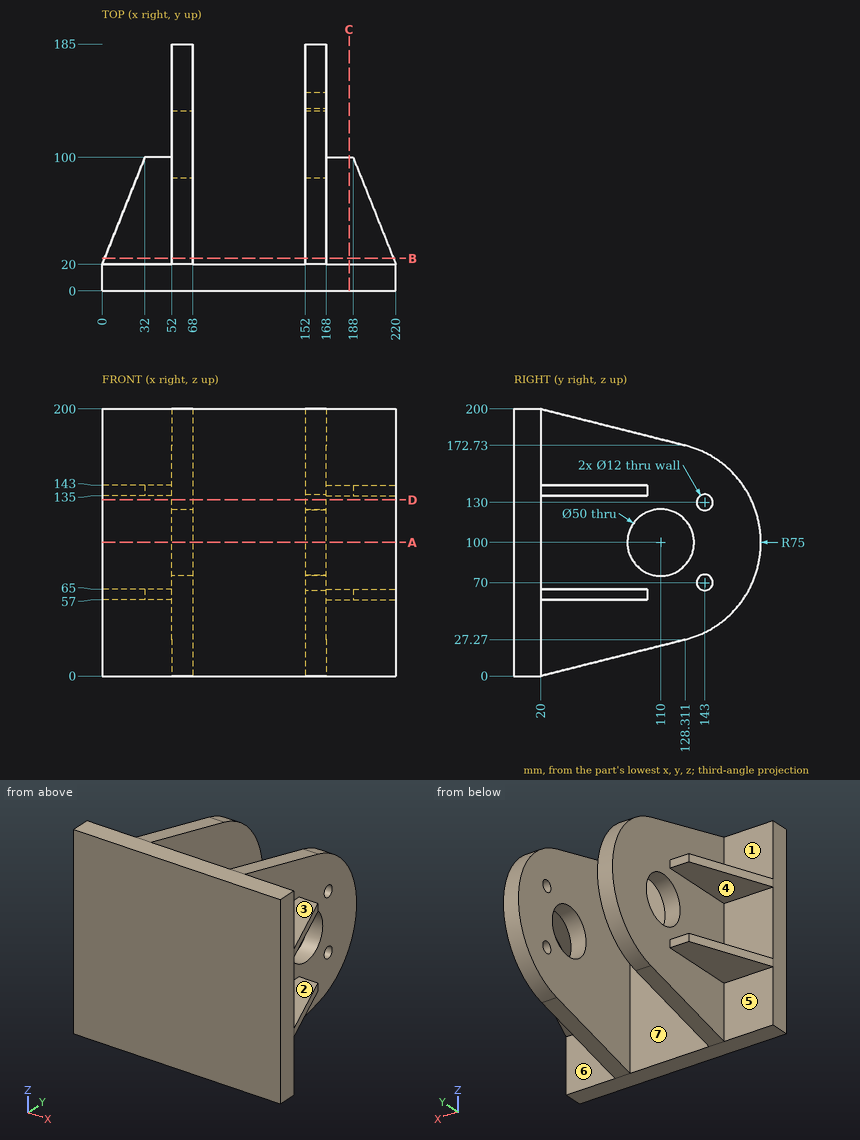
Here's the drawing with two shaded views (mm, measured from the low corner). I have some questions. A direction names the side the tool comes from. Round coordinates to 2 decimals unless told otherwise and drop trailing zeros. Loops run counter-clockwise (first coordinate to the right, second up) from the corner with the lowest first, then second, coordinate; pieces in that order, holes last. Notation, with made-up numbers: (81, -23) -> (138, -23) arc R21 cw to (138, -12) -> close; hole circle Ø8 at (-34.75, -8). An arc over 180 degrees is marked (long way). Answer as CSV lines item,"result". Start each with the question number.
1. Imagine slicing it at D-D on z = 132. Write out the boundary of the cut face in (x, y).
2. Imagine slicing it at A-A on z = 100. Write out the boundary of the cut face in (x, y), plus the area to 3 significant figures.
3. For the marked faces 1, 2, 3, 4 and 5, which set-ups out of +Z, -Z, +X, -X, +Y, -Y let a thin tool reach every point of the face, with its end or its side?
4. Imagine slicing it at C-C on x = 185. Write out the boundary of the cut face in (y, z).
5. Imagine slicing it at B-B on y = 24.5. Write out the boundary of the cut face in (x, z), plus the area to 3 significant figures.
6. I need wall thicknesses on probe 1 along X at (y, z) = (91, 54.5); probe 2 along Z at (x, y) = (176.5, 27); probe 3 along Y at (x, z) = (127.5, 146). Which ranges of each line are inside material? Lowest first, please. Write a range as from..to.
7. If we mould it in two halves opening along X, with no side actions, what happens to the marked faces 6 and 7? For each: pulls with the +X half, pulls with the -X half, needs draft (parallel to the pull), parting line crosses it, or undercut.
8. I'm going to push flat-ended pins straight in: P1, Ø6, axis at y = 49, z = 84.5, coming from the -X side; P2, Ø4, axis at x = 38.5, z = 62.5, coming from the +Y side; P3, Ø6, axis at y = 118, z = 166.5, coming from the +X side. Where does each tip first touch, or does it pass through?
Solution:
1,outline,"(0, 0) -> (220, 0) -> (220, 20) -> (168, 20) -> (168, 137.34) -> (152, 137.34) -> (152, 20) -> (68, 20) -> (68, 177.83) -> (52, 177.83) -> (52, 20) -> (0, 20) -> close; (152, 148.66) -> (168, 148.66) -> (168, 177.83) -> (152, 177.83) -> close"
2,outline,"(0, 0) -> (220, 0) -> (220, 20) -> (168, 20) -> (168, 85) -> (152, 85) -> (152, 20) -> (68, 20) -> (68, 85) -> (52, 85) -> (52, 20) -> (0, 20) -> close; (52, 135) -> (68, 135) -> (68, 185) -> (52, 185) -> close; (152, 135) -> (168, 135) -> (168, 185) -> (152, 185) -> close"
2,area,"8,080 mm²"
3,face 1,"+Z, -X, +Y"
3,face 2,"+X, +Y"
3,face 3,"+Z, +X, +Y"
3,face 4,"-X, +Y"
3,face 5,"-Z, -X, +Y"
4,outline,"(0, 0) -> (20, 0) -> (20, 57) -> (100, 57) -> (100, 65) -> (20, 65) -> (20, 135) -> (100, 135) -> (100, 143) -> (20, 143) -> (20, 200) -> (0, 200) -> close"
5,outline,"(1.8, 57) -> (52, 57) -> (52, 1.13) -> (68, 1.13) -> (68, 198.87) -> (52, 198.87) -> (52, 143) -> (1.8, 143) -> (1.8, 135) -> (52, 135) -> (52, 65) -> (1.8, 65) -> close; (152, 1.13) -> (168, 1.13) -> (168, 57) -> (218.2, 57) -> (218.2, 65) -> (168, 65) -> (168, 135) -> (218.2, 135) -> (218.2, 143) -> (168, 143) -> (168, 198.87) -> (152, 198.87) -> close"
5,area,"7,930 mm²"
6,probe 1,"52..68, 152..168"
6,probe 2,"57..65, 135..143"
6,probe 3,"0..20"
7,face 6,"needs draft"
7,face 7,"undercut"
8,P1,"x = 52"
8,P2,"y = 100"
8,P3,"x = 168"
